For this review, use the dimensioned drawing (mm, ordinates from the lowest corner) and the shaded views. Coordinates: 2 decimals unless noted, no trailing zeros. Write each loop counter-clockwise with the first axis right and the second up, starting at its lowest first coordinate (ties: lowest second). Pieces come first, ordered by that corner, then holes.
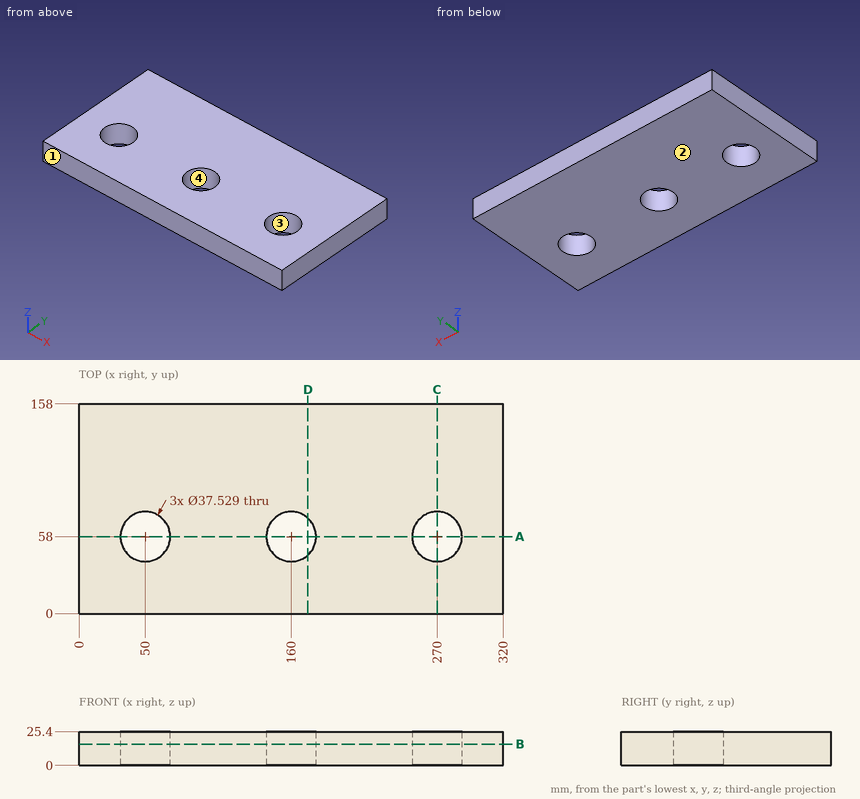
Item 1: To check wall thickness, follow line 1 along Y through (x, z) = (50, 8) (1 decimal); line 2 along X through (y, z) = (55.5, 10.75); line 3 along X through (y, z) = (54.5, 13.5) (1 decimal). State the ranges of each line that lie inside material, in increasing order.
Solved:
line 1: y = 0 to 39.2, 76.8 to 158
line 2: x = 0 to 31.4, 68.6 to 141.4, 178.6 to 251.4, 288.6 to 320
line 3: x = 0 to 31.6, 68.4 to 141.6, 178.4 to 251.6, 288.4 to 320
Item 2: Take a section at D-D, the plane x = 172.5. Write out the cut boundary in (y, z) (1 decimal).
Solved:
outline: (0, 0) - (44, 0) - (44, 25.4) - (0, 25.4) - close; (72, 0) - (158, 0) - (158, 25.4) - (72, 25.4) - close
Item 3: Take a section at B-B, the plane z = 16. Write out the cut boundary in (x, y) (1 decimal), plus the area to 3 significant figures.
Solved:
outline: (0, 0) - (320, 0) - (320, 158) - (0, 158) - close; hole circle Ø37.5 at (50, 58); hole circle Ø37.5 at (160, 58); hole circle Ø37.5 at (270, 58)
area: 47,200 mm2
Item 4: Mouldability with a two-part tool opening along Y and no side actions: class the marked faces 1, 2, 3 and 4 as pulls with the +Y half, pulls with the -Y half, needs draft (parallel to the pull), parting line crosses it, or undercut.
Solved:
face 1: pulls with the -Y half
face 2: needs draft
face 3: undercut
face 4: undercut
Item 5: Take a section at A-A, the plane y = 58. Write out the cut boundary in (x, z) (1 decimal), plus the area to 3 significant figures.
Solved:
outline: (0, 0) - (31.2, 0) - (31.2, 25.4) - (0, 25.4) - close; (68.8, 0) - (141.2, 0) - (141.2, 25.4) - (68.8, 25.4) - close; (178.8, 0) - (251.2, 0) - (251.2, 25.4) - (178.8, 25.4) - close; (288.8, 0) - (320, 0) - (320, 25.4) - (288.8, 25.4) - close
area: 5,270 mm2
Item 6: Take a section at C-C, the plane x = 270. Write out the cut boundary in (y, z) (1 decimal), plus the area to 3 significant figures.
Solved:
outline: (0, 0) - (39.2, 0) - (39.2, 25.4) - (0, 25.4) - close; (76.8, 0) - (158, 0) - (158, 25.4) - (76.8, 25.4) - close
area: 3,060 mm2
